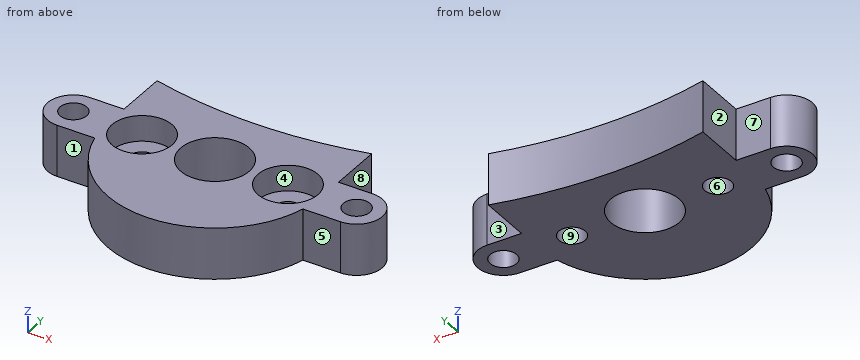
```python
from build123d import *

# Parameters (mm, degrees)
SKETCH1_R           = 1.55
SKETCH1_R_2         = 4
BOSS_EXTRUDE1_DEPTH = 6
SKETCH2_R           = 3.5
CUT_EXTRUDE1_DEPTH  = 3


with BuildPart() as part:
    # Sketch1 → Boss-Extrude1 (new body)
    with BuildSketch(Plane.XY):
        with BuildLine():
            Line((-16.5, 3), (-12.5, 3))
            Line((-12.5, 3), (-12.5, 9.132525127))
            ThreePointArc((-12.5, 9.132525127), (0, 7.619182901), (12.5, 9.132525127))
            Line((12.5, 9.132525127), (12.5, 3))
            Line((12.5, 3), (16.5, 3))
            ThreePointArc((16.5, 3), (19.5, 0), (16.5, -3))
            Line((16.5, -3), (12.1346611, -3))
            ThreePointArc((12.1346611, -3), (0, -12.5), (-12.1346611, -3))
            Line((-12.1346611, -3), (-16.5, -3))
            ThreePointArc((-16.5, -3), (-19.5, 0), (-16.5, 3))
        make_face()
        with Locations((-8.5, 0)):
            Circle(SKETCH1_R, mode=Mode.SUBTRACT)
        with Locations((8.5, 0)):
            Circle(SKETCH1_R, mode=Mode.SUBTRACT)
        Circle(SKETCH1_R_2, mode=Mode.SUBTRACT)
        with Locations((-16.5, 0)):
            Circle(SKETCH1_R, mode=Mode.SUBTRACT)
        with Locations((16.5, 0)):
            Circle(SKETCH1_R, mode=Mode.SUBTRACT)
    extrude(amount=BOSS_EXTRUDE1_DEPTH)

    # Sketch2 → Cut-Extrude1 (cut)
    with BuildSketch(Plane.XY.offset(6)):
        with Locations((-8.5, 0)):
            Circle(SKETCH2_R)
        with Locations((8.5, 0)):
            Circle(SKETCH2_R)
    extrude(amount=-CUT_EXTRUDE1_DEPTH, mode=Mode.SUBTRACT)


solid = part.part
```
Can you work these out from the model? Positions are in its coordinate system, mm. Face numbers are marked on the shaded views. A direction names the side the tool comes from. Give positions to 0.01 mm unless a question says otherwise; leave off trailing zeros. Loops run counter-clockwise (first coordinate to the right, second up) from the corner with the lowest first, then second, coordinate; pieces in that order, holes last. Notation, with made-up numbers: M 16,-26.75 L 63,-26.75 A16 cw 63,2.25 Z; hole C 54.25,63.5 d3. An arc over 180 degrees is marked long. Use one line per item in the form item = value. Start each with the question number.
(1) I'm going to push flat-ended pins straight in: P1, Ø3, axis at x = 15.5, y = 7, coming from the +Z side; P2, Ø3, axis at y = 7, z = 3.5, coming from the -X side; P3, Ø1.2, axis at x = -13.5, z = 2.5, coming from the +Y side; P4, Ø2, axis at y = -4.5, z = 4.5, coming from the -X side. Where does each tip first touch, or does it pass through?
(2) Please list where these lines run through material, in increasing order: line 1 (X direction, y = -1, z = 4.15); line 2 (X direction, y = -0.75, z = 2.85); line 3 (Y direction, x = 16.5, z = 1.6).
(3) Thinking about a two-plate mould opening in Y: for the marked faces 6, 7, 8 and 9, which applies, released by +Y, released by -Y, zero draft, split by the parting line, or undercut?
(4) I want a section at C-C, the plane x = 0. Write out the boundary of the cut face in (y, z).
(5) I want a section at D-D, the plane x = -8.5. Write out the boundary of the cut face in (y, z), and give its area (3 significant figures).
(6) On a 3-axis mill with a long thin cutter (end or side, diameter ignored), from which of +Z, -Z, +X, -X, +Y, -Y can I reach the whole of each face in a straight line? I mean the marked faces 1, 2, 3, 4 and 5. Say none if no direction works.
(7) I want a section at B-B, the plane z = 4. Write out the boundary of the cut face in (x, y), and give its area (3 significant figures).
(8) I want a section at A-A, the plane y = 0. State how many separate pieces and enclosed holes the cut face has, and give its area (3 significant figures).
Worked out:
q1.P1 = through
q1.P2 = -12.5
q1.P3 = 3
q1.P4 = -12
q2.line_1 = -19.33 to -17.68, -15.32 to -11.85, -5.15 to -3.87, 3.87 to 5.15, 11.85 to 15.32, 17.68 to 19.33
q2.line_2 = -19.4 to -17.86, -15.14 to -9.86, -7.14 to -3.93, 3.93 to 7.14, 9.86 to 15.14, 17.86 to 19.4
q2.line_3 = -3 to -1.55, 1.55 to 3
q3.face_6 = undercut
q3.face_7 = released by +Y
q3.face_8 = zero draft
q3.face_9 = undercut
q4.outline = M -12.5,0 L -4,0 L -4,6 L -12.5,6 Z; M 4,0 L 7.62,0 L 7.62,6 L 4,6 Z
q5.outline = M -9.17,0 L -1.55,0 L -1.55,3 L -3.5,3 L -3.5,6 L -9.17,6 Z; M 1.55,0 L 8.31,0 L 8.31,6 L 3.5,6 L 3.5,3 L 1.55,3 Z
q5.area = 74.6 mm²
q6.face_1 = +Z, -Z, -X, -Y
q6.face_2 = +Z, -Z, -X, +Y
q6.face_3 = +Z, -Z, +X, +Y
q6.face_4 = +Z
q6.face_5 = +Z, -Z, +X, -Y
q7.outline = M -16.5,-3 L -12.13,-3 A12.5 ccw 12.13,-3 L 16.5,-3 A3 ccw 16.5,3 L 12.5,3 L 12.5,9.13 A52.38 cw -12.5,9.13 L -12.5,3 L -16.5,3 A3 ccw Z; hole C -16.5,0 d3.1; hole C -8.5,0 d7; hole C 0,0 d8; hole C 8.5,0 d7; hole C 16.5,0 d3.1
q7.area = 383 mm²
q8.separate_pieces = 6
q8.enclosed_holes = 0
q8.area = 88.2 mm²
